Here's how the part is built. I have some questions about the finished solid (model axes, mm). Face numbers are marked on the shaded views. A direction names the side the tool comes from. Round coordinates to 2 decimals unless told otherwise and drop trailing zeros. Write each loop counter-clockwise with the first axis right and the second up, starting at its lowest first coordinate (ties: lowest second). Pieces come first, ordered by that corner, then holes. Notation, with made-up numbers: (-16, 87) -> (41, 87) arc R29 ccw to (41, 112) -> close; hole circle Ø2 at (61.5, -12). An arc over 180 degrees is marked (long way). Answer in a Markdown table with one row per item.
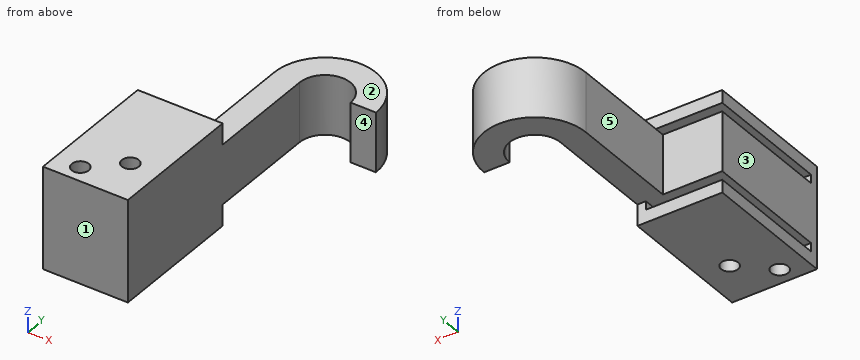
from build123d import *

# Parameters (mm, degrees)
SKETCH1_W               = 0.254
SKETCH1_H               = 25.4
SKETCH1_W_2             = 25.4
SKETCH1_H_2             = 152.4
BOSS_EXTRUDE1_DEPTH     = 76.2
SKETCH5_W               = 38.1
SKETCH5_H               = 368.3
BOSS_EXTRUDE2_DEPTH     = 44.45
SKETCH6_W               = 127
SKETCH6_H               = 203.2
BOSS_EXTRUDE3_DEPTH     = 76.2
CUT_EXTRUDE1_DEPTH      = 462.588658873
CUT_EXTRUDE1_DEPTH_BACK = 462.588658873
SKETCH7_R               = 12.7
SKETCH8_W               = 114.3
SKETCH8_H               = 190.5
CUT_EXTRUDE2_DEPTH      = 6.35


with BuildPart() as part:
    # Sketch1 → Boss-Extrude1 (new, symmetric)
    with BuildSketch(Plane.XY):
        with Locations((-25.527, 12.7)):
            Rectangle(SKETCH1_W, SKETCH1_H)
        with Locations((-12.7, 76.2)):
            Rectangle(SKETCH1_W_2, SKETCH1_H_2)
        Polygon((0, 152.4), (0, 0), (-25.4, 0), (-25.4, -25.4), (25.4, -25.4), (25.4, 177.8), (-25.4, 177.8), (-25.4, 152.4), align=None)
    extrude(amount=BOSS_EXTRUDE1_DEPTH, both=True)

    # Sketch5 → Boss-Extrude2 (add, symmetric)
    with BuildSketch(Plane.XY):
        with BuildLine():
            ThreePointArc((139.7, 342.9), (101.6, 381), (63.5, 342.9))
            Line((63.5, 342.9), (25.4, 342.9))
            ThreePointArc((25.4, 342.9), (101.6, 419.1), (177.8, 342.9))
            Line((177.8, 342.9), (139.7, 342.9))
        make_face()
        with Locations((44.45, 158.75)):
            Rectangle(SKETCH5_W, SKETCH5_H)
    extrude(amount=BOSS_EXTRUDE2_DEPTH, both=True)

    # Sketch6 → Boss-Extrude3 (add, symmetric)
    with BuildSketch(Plane.XY):
        with Locations((0, 76.2)):
            Rectangle(SKETCH6_W, SKETCH6_H)
    extrude(amount=BOSS_EXTRUDE3_DEPTH, both=True)

    # Sketch7 → Cut-Extrude1 (cut, two sides: drawn at the far end of the back side and taken through both)
    with BuildSketch(Plane.XY.offset(-CUT_EXTRUDE1_DEPTH_BACK)):
        with Locations((-25.4, 0)):
            Circle(SKETCH7_R)
        with Locations((20.32, 41.91)):
            Circle(SKETCH7_R)
    extrude(amount=CUT_EXTRUDE1_DEPTH + CUT_EXTRUDE1_DEPTH_BACK, mode=Mode.SUBTRACT)

    # Sketch8 → Cut-Extrude2 (cut, symmetric)
    with BuildSketch(Plane.XY.offset(50.8)):
        with Locations((-6.35, 82.55)):
            Rectangle(SKETCH8_W, SKETCH8_H)
    cut_extrude2 = extrude(amount=CUT_EXTRUDE2_DEPTH, both=True, mode=Mode.SUBTRACT)

    # Mirror1: Cut-Extrude2 across plane
    add(cut_extrude2.mirror(Plane.XY), mode=Mode.SUBTRACT)


solid = part.part
1) I want a section at B-B, the plane z = 33.5. List the corners of the cut face in (x, y) for me.
Response:
| item | result |
|---|---|
| outline | (-63.5, -25.4) -> (63.5, -25.4) -> (63.5, 342.9) arc R38.1 cw to (139.7, 342.9) -> (177.8, 342.9) arc R76.2 ccw to (25.4, 342.9) -> (25.4, 177.8) -> (-63.5, 177.8) -> close; hole circle Ø25.4 at (-25.4, 0); hole circle Ø25.4 at (20.32, 41.91) |
2) Which directions (+Z, -Z, +X, -X, +Y, -Y) give clear straight access to the entire face, cutting with the end or side of a thin tool? Please do the marked faces 1, 2, 3, 4 and 5.
Response:
| item | result |
|---|---|
| face 1 | +Z, -Z, +X, -X, -Y |
| face 2 | -X, +Y |
| face 3 | +Z, -Z, -X, +Y, -Y |
| face 4 | +Z, -Z, +X, -Y |
| face 5 | +Z, -Z, -X, +Y |
3) I want a section at C-C, the plane x = 20.32. List the corners of the cut face in (y, z) for me, and give its area (3 significant figures).
Response:
| item | result |
|---|---|
| outline | (-25.4, -76.2) -> (29.21, -76.2) -> (29.21, -57.15) -> (-12.7, -57.15) -> (-12.7, -44.45) -> (29.21, -44.45) -> (29.21, 44.45) -> (-12.7, 44.45) -> (-12.7, 57.15) -> (29.21, 57.15) -> (29.21, 76.2) -> (-25.4, 76.2) -> close; (54.61, -76.2) -> (177.8, -76.2) -> (177.8, -57.15) -> (54.61, -57.15) -> close; (54.61, -44.45) -> (177.8, -44.45) -> (177.8, 44.45) -> (54.61, 44.45) -> close; (54.61, 57.15) -> (177.8, 57.15) -> (177.8, 76.2) -> (54.61, 76.2) -> close |
| area | 22,900 mm^2 |
4) I want a section at A-A, the plane y = 41.91. List the corners of the cut face in (x, z) for me, and give its area (3 significant figures).
Response:
| item | result |
|---|---|
| outline | (-63.5, -76.2) -> (7.62, -76.2) -> (7.62, -57.15) -> (-63.5, -57.15) -> close; (-63.5, -44.45) -> (7.62, -44.45) -> (7.62, 44.45) -> (-63.5, 44.45) -> close; (-63.5, 57.15) -> (7.62, 57.15) -> (7.62, 76.2) -> (-63.5, 76.2) -> close; (33.02, -76.2) -> (63.5, -76.2) -> (63.5, 76.2) -> (33.02, 76.2) -> (33.02, 57.15) -> (50.8, 57.15) -> (50.8, 44.45) -> (33.02, 44.45) -> (33.02, -44.45) -> (50.8, -44.45) -> (50.8, -57.15) -> (33.02, -57.15) -> close |
| area | 13,200 mm^2 |
5) For pin 1 (8 mm diameter, centred on x = 25.5, y = 272, fed in from -Z); pin 2 (1 mm diameter, centred on y = 105, z = -36.5, fed in from +X); pin 3 (10 mm diameter, centred on x = 16.5, z = 53.5, fed in from +Y), each with a flat end and sliding along its axis, tell me the tip position at first contact or that it passes through.
Response:
| item | result |
|---|---|
| pin 1 | stops at z = -44.45 |
| pin 2 | stops at x = 63.5 |
| pin 3 | stops at y = 177.8 |
6) I need wall thicknesses on line 1 (Z direction, x = -29, y = 44); line 2 (Y direction, x = 20.32, z = 66.5); line 3 (X direction, y = 41, z = -12). Which ranges of each line are inside material? Lowest first, please. Write a range as [from, to].
Response:
| item | result |
|---|---|
| line 1 | z = [-76.2, -57.15], [-44.45, 44.45], [57.15, 76.2] |
| line 2 | y = [-25.4, 29.21], [54.61, 177.8] |
| line 3 | x = [-63.5, 7.65], [32.99, 63.5] |
7) I want a section at D-D, the plane y = 97. List the corners of the cut face in (x, z) for me, and give its area (3 significant figures).
Response:
| item | result |
|---|---|
| outline | (-63.5, -76.2) -> (63.5, -76.2) -> (63.5, 76.2) -> (-63.5, 76.2) -> (-63.5, 57.15) -> (50.8, 57.15) -> (50.8, 44.45) -> (-63.5, 44.45) -> (-63.5, -44.45) -> (50.8, -44.45) -> (50.8, -57.15) -> (-63.5, -57.15) -> close |
| area | 16,500 mm^2 |
